Autodesk Inventor part; units mm, degrees
ref_plane "YZ Plane" through (0, 0, 0) normal (1, 0, 0) x (0, 1, 0)
ref_plane "XZ Plane" through (0, 0, 0) normal (0, 1, 0) x (-1, 0, 0)
ref_plane "XY Plane" through (0, 0, 0) normal (0, 0, 1) x (1, 0, 0)
sketch "Sketch1" plane through (0, 0, 0) normal (0, 1, 0) x (-1, 0, 0)
  line L0 (173, -130.5) -> (-173, -130.5)
  line L1 (-173, -130.5) -> (-173, 130.5)
  line L2 (-173, 130.5) -> (173, 130.5)
  line L3 (173, 130.5) -> (173, -130.5)
  point P0 (0, 0)
  point P1 (173, 0)
  point P2 (0, -130.5)
  dimension "d0" = 346
  dimension "d1" = 261
extrude "Extrusion1" add sketch "Sketch1" along normal blind 8
sketch "Esboço2" plane through (0, 8, 0) normal (0, 1, 0) x (1, 0, 0)
  line L0 (173, 130.5) -> (-173, 130.5)
  line L1 (-118.5, 130.5) -> (-70.5, 130.5)
  line L2 (-70.5, 130.5) -> (-70.5, 126.5)
  line L3 (-70.5, 126.5) -> (-118.5, 126.5)
  line L4 (-118.5, 126.5) -> (-118.5, 130.5)
  line L5 (-173, 130.5) -> (-173, -130.5)
  line L6 (-24, 130.5) -> (24, 130.5)
  line L7 (24, 130.5) -> (24, 126.5)
  line L8 (24, 126.5) -> (-24, 126.5)
  line L9 (-24, 126.5) -> (-24, 130.5)
  line L10 (70.5, 130.5) -> (118.5, 130.5)
  line L11 (118.5, 130.5) -> (118.5, 126.5)
  line L12 (118.5, 126.5) -> (70.5, 126.5)
  line L13 (70.5, 126.5) -> (70.5, 130.5)
  line L14 (173, -130.5) -> (173, 130.5)
  circle A0 centre (-118.5, 126.5) radius 1
  circle A1 centre (-70.5, 126.5) radius 1
  circle A2 centre (-24, 126.5) radius 1
  circle A3 centre (24, 126.5) radius 1
  circle A4 centre (70.5, 126.5) radius 1
  circle A5 centre (118.5, 126.5) radius 1
  point P0 (0, 0)
  dimension "d4" = 48
  dimension "d5" = 4
  dimension "d6" = 54.5
  dimension "d7" = 48
  dimension "d8" = 4
  dimension "d9" = 46.5
  dimension "d10" = 4
  dimension "d11" = 48
  dimension "d12" = 46.5
  dimension "d13" = 54.5
  dimension "d14" = 2
  dimension "d15" = 2
  dimension "d16" = 2
  dimension "d17" = 2
extrude "Extrusão2" cut sketch "Esboço2" against normal blind 10
mirror "Espelhamento1" about plane through (0, 0, 0) normal (0, 0, 1) of "Extrusão2"
sketch "Esboço3" plane through (0, 0, 0) normal (0, -1, 0) x (1, 0, 0)
  line L0 (-173, 130.5) -> (-173, -130.5)
  line L1 (-173, 130.5) -> (-165, 130.5)
  line L2 (-165, 130.5) -> (-165, 77.5)
  line L3 (-165, 77.5) -> (-173, 77.5)
  line L4 (-173, 77.5) -> (-173, 130.5)
  line L5 (-165, 26.5) -> (-173, 26.5)
  line L6 (-173, 26.5) -> (-173, -26.5)
  line L7 (-173, -26.5) -> (-165, -26.5)
  line L8 (-165, -26.5) -> (-165, 26.5)
  line L9 (-173, -130.5) -> (-165, -130.5)
  line L10 (-165, -130.5) -> (-165, -77.5)
  line L11 (-165, -77.5) -> (-173, -77.5)
  line L12 (-173, -77.5) -> (-173, -130.5)
  circle A0 centre (-165, 77.5) radius 1
  circle A1 centre (-165, 26.5) radius 1
  circle A2 centre (-165, -26.5) radius 1
  circle A3 centre (-165, -77.5) radius 1
  point P0 (0, 0)
  dimension "d20" = 8
  dimension "d21" = 53
  dimension "d22" = 53
  dimension "d23" = 51
  dimension "d24" = 51
  dimension "d25" = 53
  dimension "d26" = 2
  dimension "d27" = 2
  dimension "d28" = 2
  dimension "d29" = 2
extrude "Extrusão3" cut sketch "Esboço3" against normal blind 10
mirror "Espelhamento2" about plane through (0, 0, 0) normal (1, 0, 0) of "Extrusão3"
properties part number "BASE"
Build history of the part. All positions in model axes, mm. A direction names the side the tool comes from. Round coordinates to 2 decimals unless told otherwise and drop trailing zeros. Loops run counter-clockwise (first coordinate to the right, second up) from the corner with the lowest first, then second, coordinate; pieces in that order, holes last.
Item 1: Pin check, flat tips, straight feed: P1, Ø3, axis at x = -98.5, y = 5.5, coming from the +Z side; P2, Ø3.5, axis at y = 4, z = -129.5, coming from the +X side; P3, Ø1.5, axis at y = 2.5, z = 129.5, coming from the -X side. Stop position of each tip, or through.
Item 2: Two-plate mould, pull along X, no slides. Class faces 1 (the face through (165, 4, 104)), 2 (the face through (2, 0, 2)), 3 (the face through (95, 4, -126.5)): released by +X, released by -X, zero draft, split by the parting line, or undercut.
Item 3: Saw through at A-A (z = 98.5). List the corners of the cut face in (x, y), then the cut area to 3 significant figures.
Item 4: Drill centre lines: line 1 along Z through (x, y) = (-76, 6.25); line 2 along X through (y, z) = (3.25, -8.5). Where is each one in solid material? Low to high.
Item 5: Which spindle directions (+Z, -Z, +X, -X, +Y, -Y) get a long thin tool onto all of the face, cutting with end or side? Do faces 4 (the face through (-95, 4, 126.5)), 5 (the face through (-169, 4, -77.5)), 6 (the face through (-169, 4, 77.5)). Say none if no direction does.
Worked answers:
1. P1: stops at z = 126.5
1. P2: stops at x = 165
1. P3: stops at x = -165
2. face 1: released by +X
2. face 2: zero draft
2. face 3: undercut
3. outline: (-165, 0) - (165, 0) - (165, 8) - (-165, 8) - close
3. area: 2,640 mm2
4. line 1: z = -126.5 to 126.5
4. line 2: x = -165 to 165
5. face 4: +Z, +Y, -Y
5. face 5: -Z, -X, +Y, -Y
5. face 6: +Z, -X, +Y, -Y
